from build123d import *

# Parameters (mm, degrees)
F0_R          = 3
F0_R_2        = 2.5
F1_DEPTH      = 224.6
F2_R          = 2
F3_R          = 7
F6_DEPTH      = 30
F6_DEPTH_BACK = 30
F8_DEPTH      = 30
F8_DEPTH_BACK = 30


# Not quite as in the source:
# - a feature names something its author has since deleted; it is built from what else it names


with BuildPart() as f1:
    # F0 (on Top) → F1 (new body)
    with BuildSketch(Plane.XY):
        with BuildLine():
            Line((18.15, -30), (30, -30))
            Line((30, -30), (30, -18.15))
            Line((30, -18.15), (27.5, -18.15))
            Line((27.5, -18.15), (27.5, -20.15))
            Line((27.5, -20.15), (21.5477069044, -20.15))
            ThreePointArc((21.5477069044, -20.15), (19.5, -15), (21.5477069044, -9.85))
            Line((21.5477069044, -9.85), (27.5, -9.85))
            Line((27.5, -9.85), (27.5, -11.85))
            Line((27.5, -11.85), (30, -11.85))
            Line((30, -11.85), (30, 11.85))
            Line((30, 11.85), (27.5, 11.85))
            Line((27.5, 11.85), (27.5, 9.85))
            Line((27.5, 9.85), (21.5477069044, 9.85))
            ThreePointArc((21.5477069044, 9.85), (19.5, 15), (21.5477069044, 20.15))
            Line((21.5477069044, 20.15), (27.5, 20.15))
            Line((27.5, 20.15), (27.5, 18.15))
            Line((27.5, 18.15), (30, 18.15))
            Line((30, 18.15), (30, 30))
            Line((30, 30), (18.15, 30))
            Line((18.15, 30), (18.15, 27.5))
            Line((18.15, 27.5), (20.15, 27.5))
            Line((20.15, 27.5), (20.15, 21.5477069044))
            ThreePointArc((20.15, 21.5477069044), (15, 19.5), (9.85, 21.5477069044))
            Line((9.85, 21.5477069044), (9.85, 27.5))
            Line((9.85, 27.5), (11.85, 27.5))
            Line((11.85, 27.5), (11.85, 30))
            Line((11.85, 30), (-11.85, 30))
            Line((-11.85, 30), (-11.85, 27.5))
            Line((-11.85, 27.5), (-9.85, 27.5))
            Line((-9.85, 27.5), (-9.85, 21.5477069044))
            ThreePointArc((-9.85, 21.5477069044), (-15, 19.5), (-20.15, 21.5477069044))
            Line((-20.15, 21.5477069044), (-20.15, 27.5))
            Line((-20.15, 27.5), (-18.15, 27.5))
            Line((-18.15, 27.5), (-18.15, 30))
            Line((-18.15, 30), (-30, 30))
            Line((-30, 30), (-30, 18.15))
            Line((-30, 18.15), (-27.5, 18.15))
            Line((-27.5, 18.15), (-27.5, 20.15))
            Line((-27.5, 20.15), (-21.5477069044, 20.15))
            ThreePointArc((-21.5477069044, 20.15), (-19.5, 15), (-21.5477069044, 9.85))
            Line((-21.5477069044, 9.85), (-27.5, 9.85))
            Line((-27.5, 9.85), (-27.5, 11.85))
            Line((-27.5, 11.85), (-30, 11.85))
            Line((-30, 11.85), (-30, -11.85))
            Line((-30, -11.85), (-27.5, -11.85))
            Line((-27.5, -11.85), (-27.5, -9.85))
            Line((-27.5, -9.85), (-21.5477069044, -9.85))
            ThreePointArc((-21.5477069044, -9.85), (-19.5, -15), (-21.5477069044, -20.15))
            Line((-21.5477069044, -20.15), (-27.5, -20.15))
            Line((-27.5, -20.15), (-27.5, -18.15))
            Line((-27.5, -18.15), (-30, -18.15))
            Line((-30, -18.15), (-30, -30))
            Line((-30, -30), (-18.15, -30))
            Line((-18.15, -30), (-18.15, -27.5))
            Line((-18.15, -27.5), (-20.15, -27.5))
            Line((-20.15, -27.5), (-20.15, -21.5477069044))
            ThreePointArc((-20.15, -21.5477069044), (-15, -19.5), (-9.85, -21.5477069044))
            Line((-9.85, -21.5477069044), (-9.85, -27.5))
            Line((-9.85, -27.5), (-11.85, -27.5))
            Line((-11.85, -27.5), (-11.85, -30))
            Line((-11.85, -30), (11.85, -30))
            Line((11.85, -30), (11.85, -27.5))
            Line((11.85, -27.5), (9.85, -27.5))
            Line((9.85, -27.5), (9.85, -21.5477069044))
            ThreePointArc((9.85, -21.5477069044), (15, -19.5), (20.15, -21.5477069044))
            Line((20.15, -21.5477069044), (20.15, -27.5))
            Line((20.15, -27.5), (18.15, -27.5))
            Line((18.15, -27.5), (18.15, -30))
        make_face()
        with Locations((-25, -25)):
            Circle(F0_R, mode=Mode.SUBTRACT)
        with Locations((-15, -15)):
            Circle(F0_R_2, mode=Mode.SUBTRACT)
        with Locations((25, -25)):
            Circle(F0_R, mode=Mode.SUBTRACT)
        with Locations((15, -15)):
            Circle(F0_R_2, mode=Mode.SUBTRACT)
        with Locations((-25, 25)):
            Circle(F0_R, mode=Mode.SUBTRACT)
        with Locations((-15, 15)):
            Circle(F0_R_2, mode=Mode.SUBTRACT)
        Polygon((-7, 22), (-7, 27.5), (0, 27.5), (7, 27.5), (7, 22), (10, 16), (10, 10), (16, 10), (22, 7), (27.5, 7), (27.5, 0), (27.5, -7), (22, -7), (16, -10), (10, -10), (10, -16), (7, -22), (7, -27.5), (0, -27.5), (-7, -27.5), (-7, -22), (-10, -16), (-10, -10), (-16, -10), (-22, -7), (-27.5, -7), (-27.5, 0), (-27.5, 7), (-22, 7), (-16, 10), (-10, 10), (-10, 16), align=None, mode=Mode.SUBTRACT)
        with Locations((15, 15)):
            Circle(F0_R_2, mode=Mode.SUBTRACT)
        with Locations((25, 25)):
            Circle(F0_R, mode=Mode.SUBTRACT)
    extrude(amount=F1_DEPTH)

    # F2
    f2_edges = [f1.edges().sort_by_distance(p)[0] for p in [
        (-7, 27.5, 112.3),
        (7, 27.5, 112.3),
    ]]
    fillet(f2_edges, radius=F2_R)

    # F3
    f3_edges = [f1.edges().sort_by_distance(p)[0] for p in [
        (-10, 16, 112.3),
        (10, 16, 112.3),
    ]]
    fillet(f3_edges, radius=F3_R)

    # F5 (on Right) → F6 (cut, two sides)
    with BuildSketch(Plane.YZ) as f6_sk:
        Polygon((70.3932136338, -100.3932136338), (211.6390804038, 40.8526531362), (111.24586677, 141.24586677), (-30, 0), align=None)
    extrude(amount=-F6_DEPTH, mode=Mode.SUBTRACT)
    extrude(f6_sk.sketch, amount=F6_DEPTH_BACK, mode=Mode.SUBTRACT)

    # F7 (on Front) → F8 (cut, two sides)
    with BuildSketch(Plane.XZ) as f8_sk:
        Polygon((136.0873846676, 331.4359196356), (32.0951359741, 374.5109194261), (-30, 224.6), (73.9922486935, 181.5250002095), align=None)
    extrude(amount=F8_DEPTH, mode=Mode.SUBTRACT)
    extrude(f8_sk.sketch, amount=-F8_DEPTH_BACK, mode=Mode.SUBTRACT)


solid = f1.part
Could you check a few things on this model? Use its own coordinates, in mm. A direction names the side the tool comes from. Coordinates: 2 decimals unless noted, no trailing zeros. Order: outer loops, then holes, each group sorted by start corner. A loop starts at its lowest first (then second) coordinate and runs counter-clockwise, first axis right, second up. Notation, with made-up numbers: (82, 19.25) -> (117, 19.25) arc R20 ccw to (117, 40.25) -> close; hole circle Ø8 at (-35, -13.5). An arc over 180 degrees is marked (long way). One line per question, with ' | ' between items.
Q1. If I drill on L1, parallel to X at y = -15, z = 129; L2, parallel to Y at x = 28.5, z = 165; L3, parallel to X at y = 25, z = 166, over which ranges is the centre line in solid material (lowest first)?
Return value:
L1: -19.5 to -17.5, -12.5 to -10, 10 to 12.5, 17.5 to 19.5 | L2: -30 to -18.15, -11.85 to 11.85, 18.15 to 30 | L3: -30 to -28, -22 to -20.15, -9.85 to -7, 7 to 9.85, 20.15 to 22, 28 to 30
Q2. On a 3-axis mill with a long thin cutter (end or side, diameter ignored), from which of +Z, -Z, +X, -X, +Y, -Y can I reach the whole of each face in a straight line? I mean faces 5 (the face through (-9.85, 25, 133)), 6 (the face through (11, -11, 19)). Say none if no direction works.
Return value:
face 5: +Z, -Z | face 6: -Z, +X, -X, +Y
Q3. Imagine slicing it at C-C on z = 122. State how many separate pieces and enclosed holes the cut face has, and give its area (3 significant figures).
Return value:
separate pieces: 1 | enclosed holes: 9 | area: 1,080 mm²
Q4. Thinking about a two-plate mould opening in Y: for faces 1 (the face through (25, -7, 112)), 2 (the face through (-24, 30, 141)), 3 (the face through (-30, -24, 111)), 4 (the face through (-7, -25, 107)), which applies, pulls with the +Y half, pulls with the -Y half, needs draft (parallel to the pull), parting line crosses it, or undercut?
Return value:
face 1: undercut | face 2: pulls with the +Y half | face 3: needs draft | face 4: undercut
Q5. Imagine slicing it at B-B on x = -25. Please give me the cut outline in (y, z).
Return value:
outline: (-30, 0) -> (-28, 2) -> (-28, 222.53) -> (-30, 222.53) -> close; (-22, 8) -> (-20.15, 9.85) -> (-20.15, 222.53) -> (-22, 222.53) -> close; (-9.85, 20.15) -> (-7, 23) -> (-7, 222.53) -> (-9.85, 222.53) -> close; (7, 37) -> (9.85, 39.85) -> (9.85, 222.53) -> (7, 222.53) -> close; (20.15, 50.15) -> (22, 52) -> (22, 222.53) -> (20.15, 222.53) -> close; (28, 58) -> (30, 60) -> (30, 222.53) -> (28, 222.53) -> close
Q6. I'm going to push flat-ended pins straight in: P1, Ø4, axis at y = -15.5, z = 22.5, coming from the +X side; P2, Ø1.5, axis at y = -12.5, z = 82, coming from the +X side; P3, Ø7, axis at x = -25, y = 25, coming from the -Z side; P4, Ø3, axis at x = -19, y = 17.5, coming from the -Z side. Where does each tip first touch, or does it pass through?
Return value:
P1: x = 19.93 | P2: x = 30 | P3: z = 51.5 | P4: z = 46
Q7. Imagine slicing it at A-A on x = 3. Please give me the cut outline in (y, z), and give its area (3 significant figures).
Return value:
outline: (-30, 0) -> (-27.5, 2.5) -> (-27.5, 210.93) -> (-30, 210.93) -> close; (27.5, 57.5) -> (30, 60) -> (30, 210.93) -> (27.5, 210.93) -> close | area: 905 mm²
